from build123d import *

# Parameters (mm, degrees)
BOSS_EXTRUDE1_DEPTH      = 2
BOSS_EXTRUDE1_DEPTH_BACK = 3
SKETCH1_R                = 16
SKETCH1_R_2              = 1.25
SKETCH2_R                = 5
SKETCH2_R_2              = 3
BOSS_EXTRUDE3_DEPTH      = 3
SKETCH5_R                = 2.75
CUT_EXTRUDE2_DEPTH       = 1
SKETCH6_R                = 16
SKETCH6_R_2              = 11
SKETCH6_R_3              = 1.25
BOSS_EXTRUDE4_DEPTH      = 5
SKETCH7_R                = 18
SKETCH7_R_2              = 16
BOSS_EXTRUDE5_DEPTH      = 10
SKETCH8_R                = 2
CUT_EXTRUDE3_DEPTH       = 3
SKETCH9_R                = 3.75
CUT_EXTRUDE4_DEPTH       = 2


with BuildPart() as part:
    # Sketch1 → Boss-Extrude1 (new, two sides: drawn at the far end of the back side and taken through both)
    with BuildSketch(Plane(origin=(0, 0, 0), x_dir=(1, 0, 0), z_dir=(0, 1, 0)).offset(-BOSS_EXTRUDE1_DEPTH_BACK)):
        with Locations(Location((0, 0, 0), (0, 0, 270))):
            Circle(SKETCH1_R)
        with Locations(Location((0, 0, 0), (0, 0, 270))):
            Circle(SKETCH1_R_2, mode=Mode.SUBTRACT)
        with Locations(Location((-13.5, 0, 0), (0, 0, 270))):
            Circle(SKETCH1_R_2, mode=Mode.SUBTRACT)
        with Locations(Location((-4.171729424, 12.83926297, 0), (0, 0, 270))):
            Circle(SKETCH1_R_2, mode=Mode.SUBTRACT)
        with Locations(Location((10.921729424, 7.935100906, 0), (0, 0, 270))):
            Circle(SKETCH1_R_2, mode=Mode.SUBTRACT)
        with Locations(Location((10.921729424, -7.935100906, 0), (0, 0, 270))):
            Circle(SKETCH1_R_2, mode=Mode.SUBTRACT)
        with Locations(Location((-4.171729424, -12.83926297, 0), (0, 0, 270))):
            Circle(SKETCH1_R_2, mode=Mode.SUBTRACT)
    extrude(amount=BOSS_EXTRUDE1_DEPTH + BOSS_EXTRUDE1_DEPTH_BACK)

    # Sketch2 → Boss-Extrude3 (add)
    with BuildSketch(Plane(origin=(0, 2, 0), x_dir=(1, 0, 0), z_dir=(0, 1, 0))):
        with Locations(Location((0, 0, 0), (0, 0, 270))):
            Circle(SKETCH2_R)
        with Locations(Location((0, 0, 0), (0, 0, 270))):
            Circle(SKETCH2_R_2, mode=Mode.SUBTRACT)
    extrude(amount=BOSS_EXTRUDE3_DEPTH)

    # Sketch5 → Cut-Extrude2 (cut)
    with BuildSketch(Plane.XZ.offset(3)):
        with Locations(Location((0, 0, 0), (0, 0, 270))):
            Circle(SKETCH5_R)
    extrude(amount=-CUT_EXTRUDE2_DEPTH, mode=Mode.SUBTRACT)

    # Sketch6 → Boss-Extrude4 (add)
    with BuildSketch(Plane.XZ.offset(3)):
        with Locations(Location((0, 0, 0), (0, 0, 90))):
            Circle(SKETCH6_R)
        with Locations(Location((0, 0, 0), (0, 0, 270))):
            Circle(SKETCH6_R_2, mode=Mode.SUBTRACT)
        with Locations(Location((-13.5, 0, 0), (0, 0, 90))):
            Circle(SKETCH6_R_3, mode=Mode.SUBTRACT)
        with Locations(Location((-4.171729424, 12.83926297, 0), (0, 0, 90))):
            Circle(SKETCH6_R_3, mode=Mode.SUBTRACT)
        with Locations(Location((10.921729424, 7.935100906, 0), (0, 0, 90))):
            Circle(SKETCH6_R_3, mode=Mode.SUBTRACT)
        with Locations(Location((10.921729424, -7.935100906, 0), (0, 0, 90))):
            Circle(SKETCH6_R_3, mode=Mode.SUBTRACT)
        with Locations(Location((-4.171729424, -12.83926297, 0), (0, 0, 90))):
            Circle(SKETCH6_R_3, mode=Mode.SUBTRACT)
    extrude(amount=BOSS_EXTRUDE4_DEPTH)

    # Sketch7 → Boss-Extrude5 (add)
    with BuildSketch(Plane(origin=(0, 2, 0), x_dir=(1, 0, 0), z_dir=(0, 1, 0))):
        with Locations(Location((0, 0, 0), (0, 0, 270))):
            Circle(SKETCH7_R)
        Circle(SKETCH7_R_2, mode=Mode.SUBTRACT)
    extrude(amount=-BOSS_EXTRUDE5_DEPTH)

    # Sketch8 → Cut-Extrude3 (cut)
    with BuildSketch(Plane.XZ.offset(2)):
        with Locations(Location((0, 0, 0), (0, 0, 270))):
            Circle(SKETCH8_R)
    extrude(amount=-CUT_EXTRUDE3_DEPTH, mode=Mode.SUBTRACT)

    # Sketch9 → Cut-Extrude4 (cut)
    with BuildSketch(Plane.XZ.offset(3)):
        with Locations(Location((0, 0, 0), (0, 0, 270))):
            Circle(SKETCH9_R)
    extrude(amount=-CUT_EXTRUDE4_DEPTH, mode=Mode.SUBTRACT)


solid = part.part
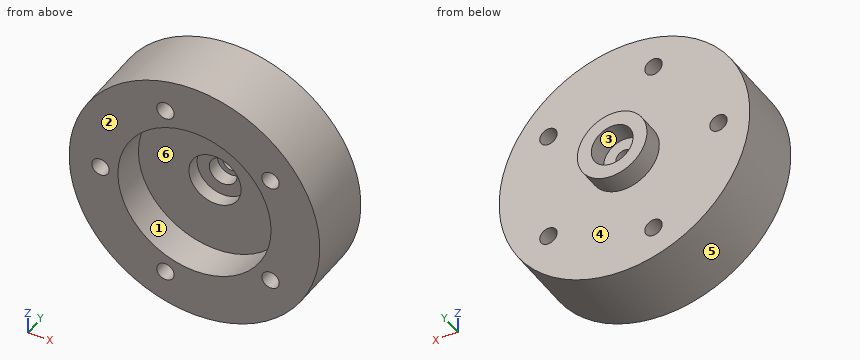
The listing builds one solid part. Answer for the finished solid, in the listing's coordinates (mm). Face numbers are marked on the shaded views. A direction names the side the tool comes from. Coordinates: 2 decimals unless noted, no trailing zeros. Write each loop counter-clockwise with the first axis right and the second up, starting at its lowest first coordinate (ties: lowest second). Pieces come first, ordered by that corner, then holes. Notation, with made-up numbers: (17.5, 55) -> (34.5, 55) arc R37 ccw to (34.5, 94) -> close; hole circle Ø5 at (61, -21.5). An arc over 180 degrees is marked (long way). One line per question, with ' | ' between items.
1. Which of the six approach directions +Z, -Z, +X, -X, +Y, -Y give full straight-line access (tool end or side, diameter ignored) to the marked faces 1, 2 and 3?
Verdict:
face 1: -Y | face 2: +Z, -Z, +X, -X, -Y | face 3: +Y
2. Section C-C (y = 3.75) is taken. Determine the outline of the cut face in (x, z).
Verdict:
outline: circle Ø10 at (0, 0); hole circle Ø6 at (0, 0)
3. Straight lines are drawn through the part: line 1 (X direction, y = -0.5, z = 0); line 2 (X direction, y = 3.3, z = 0); line 3 (Z direction, x = 11, y = -2.5). For each, find the intervals that lie inside material, in ascending order.
Verdict:
line 1: x = -18 to -14.75, -12.25 to -2, 2 to 18 | line 2: x = -5 to -3, 3 to 5 | line 3: z = -14.25 to -9.18, -6.69 to 6.69, 9.18 to 14.25
4. Section B-B (x = 0) is taken. Determine the outline of the cut face in (y, z).
Verdict:
outline: (-8, -18) -> (2, -18) -> (2, -5) -> (5, -5) -> (5, -3) -> (2, -3) -> (2, -1.25) -> (1, -1.25) -> (1, -2) -> (-1, -2) -> (-1, -3.75) -> (-3, -3.75) -> (-3, -11) -> (-8, -11) -> close; (-8, 11) -> (-3, 11) -> (-3, 3.75) -> (-1, 3.75) -> (-1, 2) -> (1, 2) -> (1, 1.25) -> (2, 1.25) -> (2, 3) -> (5, 3) -> (5, 5) -> (2, 5) -> (2, 18) -> (-8, 18) -> close
5. Section A-A (z = 0) is taken. State how many separate pieces and enclosed holes the cut face has, and give its area (4 significant figures).
Verdict:
separate pieces: 3 | enclosed holes: 0 | area: 211.5 mm^2
6. Given pin 1 Ø1.5 at (y, z) = (1.5, -7) entering from -X; pin 2 Ø5 at (x, z) = (0, 0) entering from +Y; pin 3 Ø10 at (x, z) = (0, 0) entering from -Y; pin 4 Ø2 at (x, z) = (-13.5, 0) entering from -Y, each flat-ended and moving along its own axis, determine where each tip first touches the part or whether it passes through.
Verdict:
pin 1: stops at x = -16.88 | pin 2: stops at y = 2 | pin 3: stops at y = -3 | pin 4: passes through
7. Section D-D (y = -4.5) is taken. Determine the outline of the cut face in (x, z), and give its area (3 significant figures).
Verdict:
outline: circle Ø36 at (0, 0); hole circle Ø2.5 at (-13.5, 0); hole circle Ø22 at (0, 0); hole circle Ø2.5 at (-4.17, -12.84); hole circle Ø2.5 at (-4.17, 12.84); hole circle Ø2.5 at (10.92, -7.94); hole circle Ø2.5 at (10.92, 7.94) | area: 613 mm^2
8. For a pull along Z with two mould halves and no side action, classify the marked faces 4, 5 and 6 as released by +Z, released by -Z, zero draft, split by the parting line, or undercut.
Verdict:
face 4: zero draft | face 5: split by the parting line | face 6: undercut
